Build history of the part. All positions in model axes, mm. Face numbers are marked on the shaded views. A direction names the side the tool comes from. Give positions to 0.01 mm unless a question says otherwise; leave off trailing zeros. Loops run counter-clockwise (first coordinate to the right, second up) from the corner with the lowest first, then second, coordinate; pieces in that order, holes last.
1) Two-plate mould, pull along Y, no slides. Class the marked faces 1, 2 and 3: +Y half, -Y half, draft (parallel to the pull), parting line (faces both ways), or undercut.
2) Band-saw the part on B-B on y = 6.5. List the corners of the cut face in (x, z), then the cut area to 3 significant figures.
3) Wall check: line 1 (Z direction, x = -2.5, y = 20.35); line 2 (Y direction, x = 26, z = 8.75); line 3 (X direction, y = 25.5, z = 11). Give the ranges that are in metal, low to high.
4) Flat gauge pins, fed straight in: P1, Ø1.5, axis at y = 14.5, z = 6, coming from the -X side; P2, Ø1, axis at x = 24, y = 7.5, coming from the +Z side; P3, Ø3, axis at y = 14, z = 4.5, coming from the +X side. Where does each tip first touch, or does it go through?
5) 3-axis set-ups, long thin cutter, end or side, ignore diameter. For the marked faces 4, 5 and 6: which of +Z, -Z, +X, -X, +Y, -Y reach the whole face in a straight line?
6) Band-saw the part on C-C on z = 9.85. List the corners of the cut face in (x, y).
7) Band-saw the part on D-D on x = -2.5. List the corners of the cut face in (y, z).
8) Band-saw the part on A-A on x = 25.5. List the corners of the cut face in (y, z).
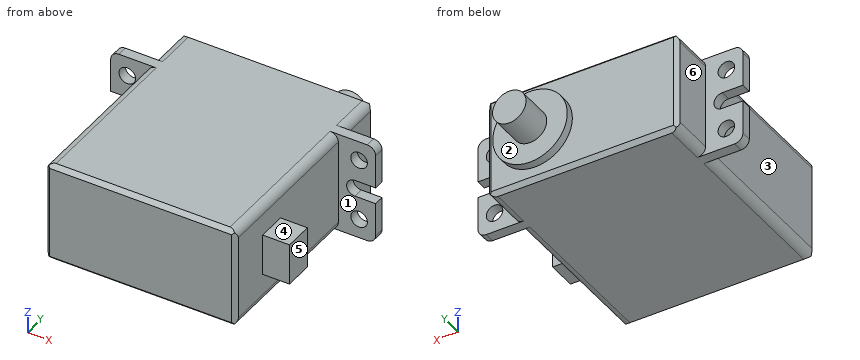
```python
from build123d import *

# Parameters (mm, degrees)
ESQUISSE1_W             = 23
ESQUISSE1_H             = 26.8
BOSS_EXTRU_1_DEPTH      = 12.2
ESQUISSE2_W             = 32
ESQUISSE2_H             = 1.25
BOSS_EXTRU_2_DEPTH      = 12.2
ESQUISSE3_R             = 4.5
BOSS_EXTRU_3_DEPTH      = 1
ESQUISSE4_R             = 2.025
BOSS_EXTRU_4_DEPTH      = 4.05
ESQUISSE5_W             = 5
ESQUISSE5_H             = 3.5
BOSS_EXTRU_5_DEPTH      = 3.25
ESQUISSE7_R             = 1
ENL_V_MAT_EXTRU_1_DEPTH = 1.25
CHANFREIN1_SIZE         = 0.5
CONG_1_R                = 1
CONG_2_R                = 1


with BuildPart() as part:
    # Esquisse1 → Boss.-Extru.1 (new body)
    with BuildSketch(Plane.XY):
        with Locations((11.5, 13.4)):
            Rectangle(ESQUISSE1_W, ESQUISSE1_H)
    extrude(amount=BOSS_EXTRU_1_DEPTH)

    # Esquisse2 → Boss.-Extru.2 (add)
    with BuildSketch(Plane.XY.offset(12.2)):
        with Locations((11.5, 20.675)):
            Rectangle(ESQUISSE2_W, ESQUISSE2_H)
    extrude(amount=-BOSS_EXTRU_2_DEPTH)

    # Esquisse3 → Boss.-Extru.3 (add)
    with BuildSketch(Plane(origin=(0, 26.8, 0), x_dir=(1, 0, 0), z_dir=(0, 1, 0))):
        with Locations(Location((17.2, -6.1, 0), (0, 0, 90))):
            Circle(ESQUISSE3_R)
    extrude(amount=BOSS_EXTRU_3_DEPTH)

    # Esquisse4 → Boss.-Extru.4 (add)
    with BuildSketch(Plane(origin=(0, 27.8, 0), x_dir=(1, 0, 0), z_dir=(0, 1, 0))):
        with Locations(Location((17.2, -6.1, 0), (0, 0, 270))):
            Circle(ESQUISSE4_R)
    extrude(amount=BOSS_EXTRU_4_DEPTH)

    # Esquisse5 → Boss.-Extru.5 (add)
    with BuildSketch(Plane(origin=(23, 0, 0), x_dir=(0, 0, -1), z_dir=(1, 0, 0))):
        with Locations((-6.1, 6.99)):
            Rectangle(ESQUISSE5_W, ESQUISSE5_H)
    extrude(amount=BOSS_EXTRU_5_DEPTH)

    # Esquisse7 → Enlèv. mat.-Extru.1 (cut)
    with BuildSketch(Plane(origin=(0, 21.3, 0), x_dir=(1, 0, 0), z_dir=(0, 1, 0))):
        with Locations(Location((25.5, -2.35, 0), (0, 0, 180))):
            Circle(ESQUISSE7_R)
        with Locations(Location((25.5, -9.85, 0), (0, 0, 180))):
            Circle(ESQUISSE7_R)
        with Locations((-2.5, -9.85)):
            Circle(ESQUISSE7_R)
        with Locations((-2.5, -2.35)):
            Circle(ESQUISSE7_R)
        with BuildLine():
            Line((30, -7.1), (25, -7.1))
            ThreePointArc((25, -7.1), (24, -6.1), (25, -5.1))
            Line((25, -5.1), (30, -5.1))
            ThreePointArc((30, -5.1), (31, -6.1), (30, -7.1))
        make_face()
        with BuildLine():
            Line((-7, -5.1), (-2, -5.1))
            ThreePointArc((-2, -5.1), (-1, -6.1), (-2, -7.1))
            Line((-2, -7.1), (-7, -7.1))
            ThreePointArc((-7, -7.1), (-8, -6.1), (-7, -5.1))
        make_face()
    extrude(amount=-ENL_V_MAT_EXTRU_1_DEPTH, mode=Mode.SUBTRACT)

    # Chanfrein1
    chanfrein1_edges = [part.edges().sort_by_distance(p)[0] for p in [
        (11.5, 26.8, 12.2),
        (11.5, 26.8, 0),
        (11.5, 0, 0),
        (11.5, 0, 12.2),
        (0, 26.8, 6.1),
        (23, 26.8, 6.1),
        (23, 0, 6.1),
        (0, 0, 6.1),
    ]]
    chamfer(chanfrein1_edges, length=CHANFREIN1_SIZE)

    # Congé1
    cong_1_edges = [part.edges().sort_by_distance(p)[0] for p in [
        (23, 10.275, 12.2),
        (0, 10.275, 0),
        (23, 10.275, 0),
        (0, 23.8, 12.2),
        (23, 23.8, 0),
        (0, 23.8, 0),
        (0, 10.275, 12.2),
        (23, 23.8, 12.2),
        (23, 10.275, 0),
        (0, 10.275, 0),
        (23, 10.275, 12.2),
        (0, 10.275, 12.2),
        (0, 10.275, 0),
        (23, 10.275, 0),
        (23, 10.275, 12.2),
        (0, 10.275, 12.2),
    ]]
    fillet(cong_1_edges, radius=CONG_1_R)

    # Congé2
    cong_2_edges = [part.edges().sort_by_distance(p)[0] for p in [
        (-4.5, 20.675, 12.2),
        (27.5, 20.675, 12.2),
        (27.5, 20.675, 0),
        (-4.5, 20.675, 0),
    ]]
    fillet(cong_2_edges, radius=CONG_2_R)


solid = part.part
```
Findings below:
1. face 1: undercut
1. face 2: +Y half
1. face 3: draft
2. outline: (0, 1) arc R1 ccw to (1, 0) - (22, 0) arc R1 ccw to (23, 1) - (23, 3.6) - (26.25, 3.6) - (26.25, 8.6) - (23, 8.6) - (23, 11.2) arc R1 ccw to (22, 12.2) - (1, 12.2) arc R1 ccw to (0, 11.2) - close
2. area: 296 mm2
3. line 1: z = 0 to 1.35, 3.35 to 5.1, 7.1 to 8.85, 10.85 to 12.2
3. line 2: y = 20.05 to 21.3
3. line 3: x = 0 to 23
4. P1: stops at x = 0
4. P2: stops at z = 8.6
4. P3: stops at x = 23
5. face 4: +Z, +X, -Y
5. face 5: +Z, -Z, +X, -Y
5. face 6: +Z, -Z, -X, +Y
6. outline: (-4.5, 20.05) - (-3.5, 20.05) - (-3.5, 21.3) - (-4.5, 21.3) - close; (-1.5, 20.05) - (0, 20.05) - (0, 0.5) - (0.5, 0) - (22.5, 0) - (23, 0.5) - (23, 20.05) - (24.5, 20.05) - (24.5, 21.3) - (23, 21.3) - (23, 26.3) - (22.5, 26.8) - (19.69, 26.8) - (19.69, 27.8) - (14.71, 27.8) - (14.71, 26.8) - (0.5, 26.8) - (0, 26.3) - (0, 21.3) - (-1.5, 21.3) - close; (26.5, 20.05) - (27.5, 20.05) - (27.5, 21.3) - (26.5, 21.3) - close
7. outline: (20.05, 0) - (21.3, 0) - (21.3, 1.35) - (20.05, 1.35) - close; (20.05, 3.35) - (21.3, 3.35) - (21.3, 5.1) - (20.05, 5.1) - close; (20.05, 7.1) - (21.3, 7.1) - (21.3, 8.85) - (20.05, 8.85) - close; (20.05, 10.85) - (21.3, 10.85) - (21.3, 12.2) - (20.05, 12.2) - close
8. outline: (5.24, 3.6) - (8.74, 3.6) - (8.74, 8.6) - (5.24, 8.6) - close; (20.05, 0) - (21.3, 0) - (21.3, 1.35) - (20.05, 1.35) - close; (20.05, 3.35) - (21.3, 3.35) - (21.3, 5.1) - (20.05, 5.1) - close; (20.05, 7.1) - (21.3, 7.1) - (21.3, 8.85) - (20.05, 8.85) - close; (20.05, 10.85) - (21.3, 10.85) - (21.3, 12.2) - (20.05, 12.2) - close
